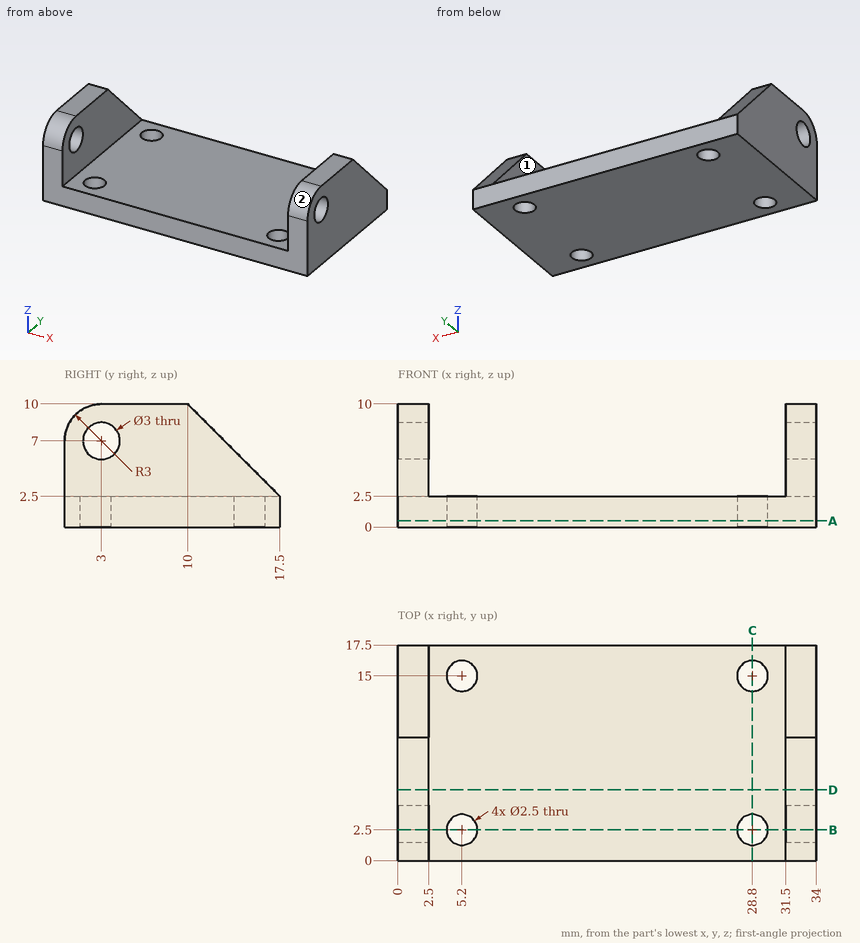
Check sheet for the drawn part. Datum: minimum x, y, z corner. Units: mm. A direction names the side the tool comes from. Round coordinates to 2 decimals unless told otherwise and drop trailing zeros. Loops run counter-clockwise (first coordinate to the right, second up) from the corner with the lowest first, then second, coordinate; pieces in that order, holes last. Notation, with made-up numbers: (-14, 60) - (38, 60) arc R18 cw to (38, 84) - close; hole circle Ø10 at (68, 67). An arc over 180 degrees is marked (long way). Write each question's results on one line, items separated by ' | '. Start each with the question number.
Q1. Cross-section at C-C on x = 28.8. Enter the section's corners in (y, z).
Q2. Access from +Z, -Z, +X, -X, +Y, -Y to the whole of each face (thin tool, end or side, straight path). Record for the marked faces 1 and 2.
Q3. Cross-section at D-D on y = 5.75. Enter the section's corners in (x, z).
Q4. Cross-section at B-B on y = 2.5. Enter the section's corners in (x, z).
Q5. Gauge pin test, flat ends, axial feed: P1, Ø2.5, axis at y = 3, z = 7, coming from the +X side; P2, Ø5, axis at x = 12.5, y = 10.5, coming from the +Z side. Record the tip position at first contact, or that the pin passes through.
Q6. Thickness scan on line 1 (Y direction, x = 28.8, z = 0.8); line 2 (Y direction, x = 29.5, z = 0.5); line 3 (X direction, y = 10.5, z = 8.75). Record the ranges inside material, lowest first. Write a range as [from, to].
Q7. Cross-section at A-A on z = 0.5. Enter the section's corners in (x, y).
Answers below:
1) outline: (0, 0) - (1.25, 0) - (1.25, 2.5) - (0, 2.5) - close; (3.75, 0) - (13.75, 0) - (13.75, 2.5) - (3.75, 2.5) - close; (16.25, 0) - (17.5, 0) - (17.5, 2.5) - (16.25, 2.5) - close
2) face 1: +Z, +Y, -Y | face 2: +Z, +X, -X, -Y
3) outline: (0, 0) - (34, 0) - (34, 10) - (31.5, 10) - (31.5, 2.5) - (2.5, 2.5) - (2.5, 10) - (0, 10) - close
4) outline: (0, 0) - (3.95, 0) - (3.95, 2.5) - (2.5, 2.5) - (2.5, 5.59) - (0, 5.59) - close; (0, 8.41) - (2.5, 8.41) - (2.5, 9.96) - (0, 9.96) - close; (6.45, 0) - (27.55, 0) - (27.55, 2.5) - (6.45, 2.5) - close; (30.05, 0) - (34, 0) - (34, 5.59) - (31.5, 5.59) - (31.5, 2.5) - (30.05, 2.5) - close; (31.5, 8.41) - (34, 8.41) - (34, 9.96) - (31.5, 9.96) - close
5) P1: passes through | P2: stops at z = 2.5
6) line 1: y = [0, 1.25], [3.75, 13.75], [16.25, 17.5] | line 2: y = [0, 1.46], [3.54, 13.96], [16.04, 17.5] | line 3: x = [0, 2.5], [31.5, 34]
7) outline: (0, 0) - (34, 0) - (34, 17.5) - (0, 17.5) - close; hole circle Ø2.5 at (5.2, 2.5); hole circle Ø2.5 at (5.2, 15); hole circle Ø2.5 at (28.8, 2.5); hole circle Ø2.5 at (28.8, 15)
